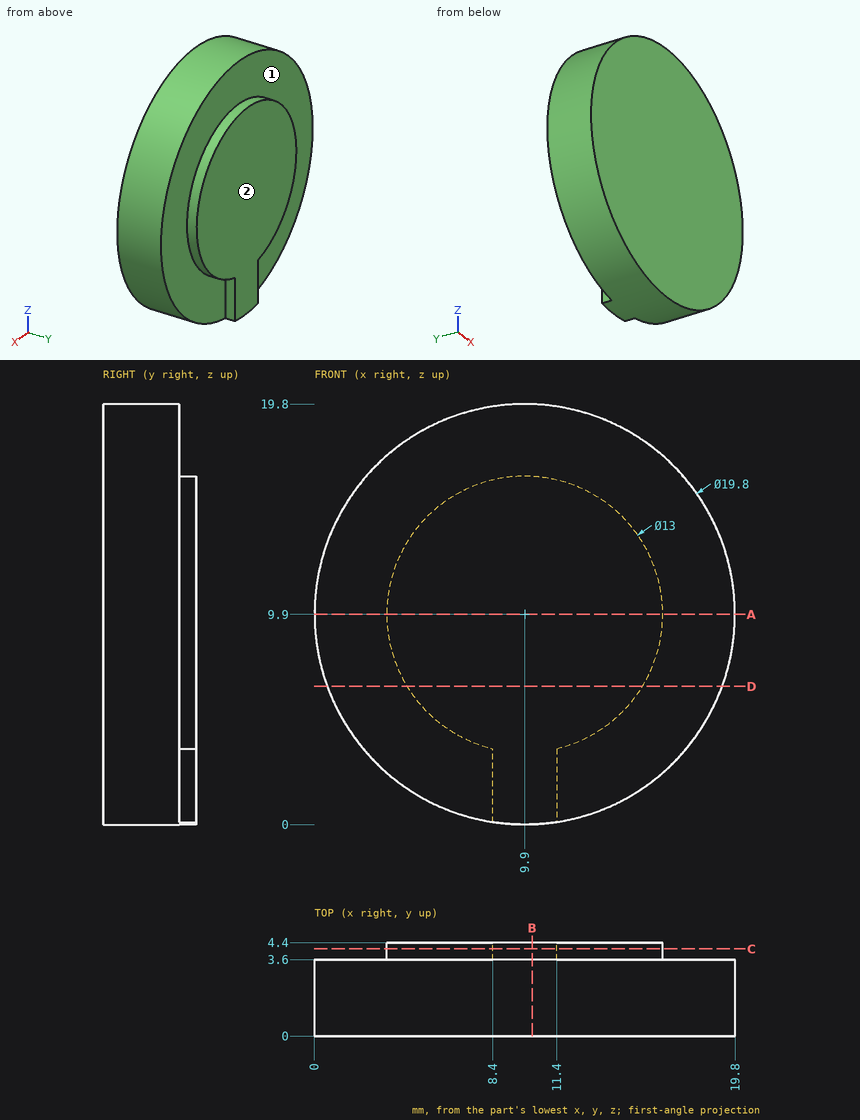
Answer from the drawing. Dimensions are ordinates in mm from the lowest x, y and z of the part. A direction names the side the tool comes from. Round coordinates to 2 decimals unless told otherwise and drop trailing zeros. Order: outer loops, then holes, each group sorted by start corner. A loop starts at its lowest first (then second) coordinate and runs counter-clockwise, first axis right, second up.
1) Straight lines are drawn through the part: L1, parallel to Y at x = 13, z = 18.75; L2, parallel to X at y = 1.45, z = 14.5; L3, parallel to Z at x = 12.75, y = 3.3. For each, find the intervals that lie inside material, in ascending order.
2) For the marked faces 1 and 2, determine the directions among +Z, -Z, +X, -X, +Y, -Y from which every point of the face is accessible in a straight line to the end or side of a thin tool.
3) Flat-ended cylindrical pins translate along their axes: pin 1 (1.5 mm diameter, centred on x = 12, y = 3, fed in from +Z); pin 2 (2 mm diameter, centred on y = 0.5, z = 12, fed in from -X); pin 3 (1 mm diameter, centred on x = 5, y = 2.5, fed in from +Z). Find the tip coordinate at first contact, or state that the pin passes through.
4) The part is cut by section C-C on y = 4.1. Write down the section's boundary in (x, z), plus the area to 3 significant figures.
5) The part is cut by section A-A on z = 9.9. Write down the section's boundary in (x, y), plus the area to 3 significant figures.
6) The part is cut by section D-D on z = 6.5. Write down the section's boundary in (x, y), plus the area to 3 significant figures.
7) The part is cut by section B-B on x = 10.25. Write down the section's boundary in (y, z), plus the area to 3 significant figures.
Resolved:
1. L1: y = 0 to 3.6
1. L2: x = 1.13 to 18.67
1. L3: z = 0.42 to 19.38
2. face 1: +Y
2. face 2: +Z, -Z, +X, -X, +Y
3. pin 1: stops at z = 19.71
3. pin 2: stops at x = 0.06
3. pin 3: stops at z = 18.77
4. outline: (8.4, 0.11) arc R9.9 ccw to (11.4, 0.11) - (11.4, 3.58) arc R6.5 ccw (long way) to (8.4, 3.58) - close
4. area: 143 mm2
5. outline: (0, 0) - (19.8, 0) - (19.8, 3.6) - (16.4, 3.6) - (16.4, 4.4) - (3.4, 4.4) - (3.4, 3.6) - (0, 3.6) - close
5. area: 81.7 mm2
6. outline: (0.6, 0) - (19.2, 0) - (19.2, 3.6) - (15.44, 3.6) - (15.44, 4.4) - (4.36, 4.4) - (4.36, 3.6) - (0.6, 3.6) - close
6. area: 75.8 mm2
7. outline: (0, 0.01) - (4.4, 0.01) - (4.4, 16.39) - (3.6, 16.39) - (3.6, 19.79) - (0, 19.79) - close
7. area: 84.3 mm2
